Could you check a few things on this drawing? It's one solid part, dimensions in mm from its lowest x, y, z. A direction names the side the tool comes from. Give positions to 0.01 mm unless a question says otherwise; leave off trailing zeros. Order: outer loops, then holes, each group sorted by start corner. A loop starts at its lowest first (then second) coordinate and runs counter-clockwise, first axis right, second up.
Item 1: Which directions (+Z, -Z, +X, -X, +Y, -Y) give clear straight access to the entire face, cutting with the end or side of a thin tool? Please do the marked faces 1 and 2.
Item 2: I want a section at C-C, the plane y = 170. Write out the boundary of the cut face in (x, z), then the cut area to 3 significant figures.
Item 3: I want a section at B-B, the plane z = 85. Write out the boundary of the cut face in (x, y).
Item 4: I'm going to push flat-ended pins straight in: pin 1 Ø6 at (y, z) = (8.5, 84) entering from +X; pin 2 Ø2 at (x, y) = (17.5, 98.5) entering from -Z; pin 3 Ø2 at (x, z) = (13, 86) entering from -Y. Where does each tip first touch, or does it pass through?
Item 5: I want a section at A-A, the plane x = 15.5. Write out the boundary of the cut face in (y, z).
Item 6: If I drill on line 1 along Z through (x, y) = (15, 170); line 2 along X through (y, z) = (8, 57); line 3 along Y through (x, z) = (18.75, 135.5), over which ranges is the centre line in solid material (lowest first)?
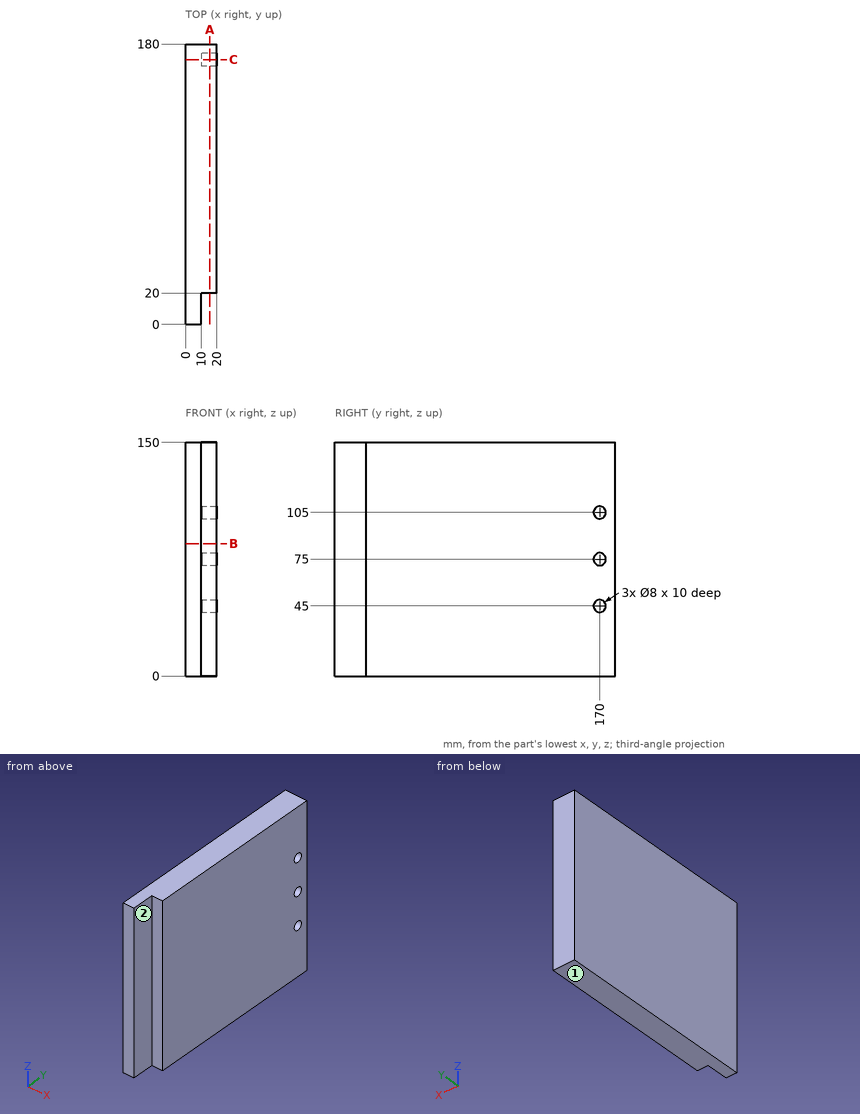
Results list:
1. face 1: -Z, +X, -X, +Y, -Y
1. face 2: +Z, -Z, +X, -Y
2. outline: (0, 0) - (20, 0) - (20, 41) - (10, 41) - (10, 49) - (20, 49) - (20, 71) - (10, 71) - (10, 79) - (20, 79) - (20, 101) - (10, 101) - (10, 109) - (20, 109) - (20, 150) - (0, 150) - close
2. area: 2,760 mm2
3. outline: (0, 0) - (10, 0) - (10, 20) - (20, 20) - (20, 180) - (0, 180) - close
4. pin 1: stops at x = 10
4. pin 2: stops at z = 0
4. pin 3: stops at y = 20
5. outline: (20, 0) - (180, 0) - (180, 150) - (20, 150) - close; hole circle Ø8 at (170, 45); hole circle Ø8 at (170, 75); hole circle Ø8 at (170, 105)
6. line 1: z = 0 to 41, 49 to 71, 79 to 101, 109 to 150
6. line 2: x = 0 to 10
6. line 3: y = 20 to 180
